Input: dimensioned drawing with shaded views. Units: mm. Origin: part minimum x, y, z. Round coordinates to 2 decimals unless told otherwise and drop trailing zeros. Loops run counter-clockwise (first coordinate to the right, second up) from the corner with the lowest first, then second, coordinate; pieces in that order, holes last. Notation, with made-up numbers: M 29,44 L 60,44 A20 cw 60,67 Z; hole C 56.5,62.5 d5. An arc over 180 degrees is marked long. Return JSON: item names as keys, results as strings.
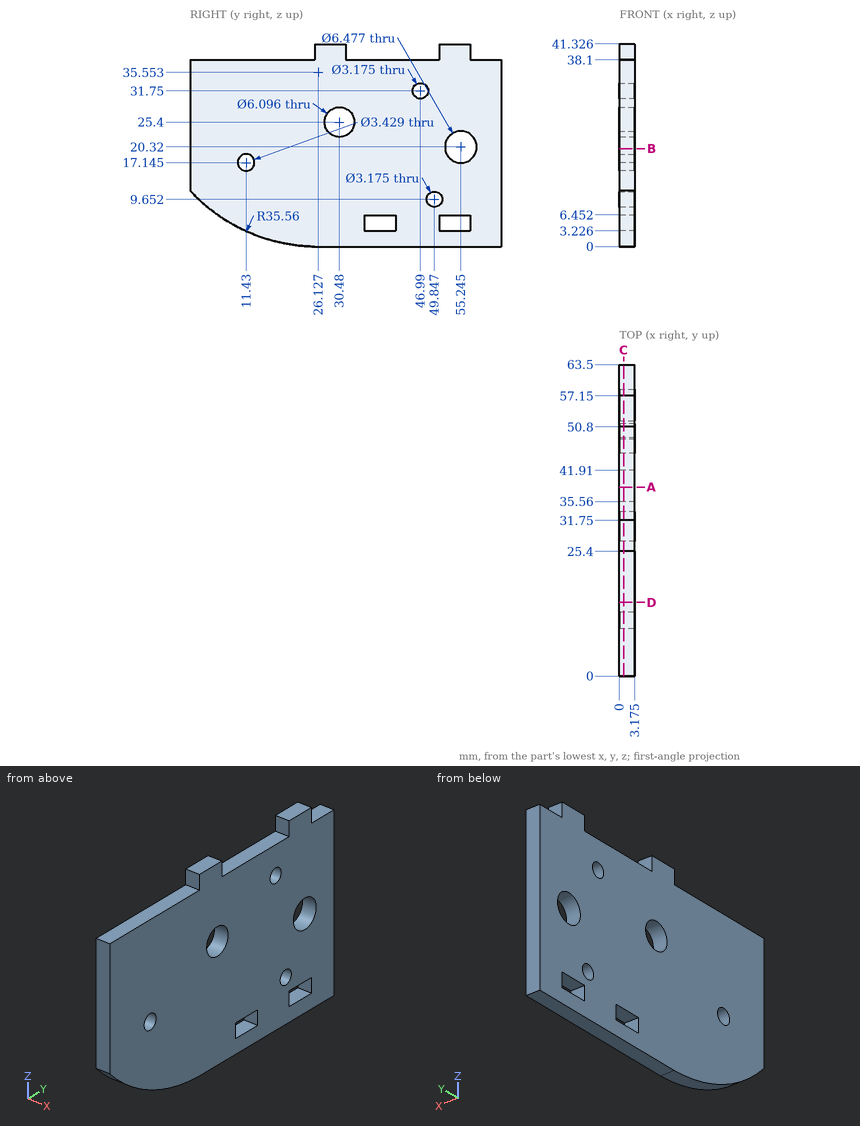
Q1. Section query C-C (x = 0.85). State how many separate pieces and enclosed holes the cut face has, plus the area to 3 significant figures.
Determined:
{"separate pieces": "1", "enclosed holes": "7", "area": "2,240 mm^2"}
Q2. Material intervals for L1, parallel to Y at x = 0.75, z = 31.75; L2, parallel to Y at x = 1.5, z = 17; L3, parallel to Z at x = 1.9, y = 31 (1 decimal), sorted ascending.
Determined:
{"L1": "y = 0 to 45.4, 48.58 to 63.5", "L2": "y = 0 to 9.72, 13.14 to 63.5", "L3": "z = 0 to 22.4, 28.4 to 41.3"}
Q3. Section query D-D (y = 15). Output: boundary loops of the cut face in (x, z) (1 decimal).
Determined:
{"outline": "M 0,1.8 L 3.2,1.8 L 3.2,38.1 L 0,38.1 Z"}
Q4. Section query B-B (z = 20). Output: boundary loops of the cut face in (x, y) (1 decimal).
Determined:
{"outline": "M 0,0 L 3.2,0 L 3.2,52 L 0,52 Z; M 0,58.5 L 3.2,58.5 L 3.2,63.5 L 0,63.5 Z"}
Q5. Pin query (flat end, axial travel): pin 1 (1.6 mm diameter, centred on x = 2, z = 40, fed in from -Y); pin 2 (1.6 mm diameter, centred on x = 1.5, y = 60.5, fed in from +Z). Return the tip coordinate at first contact, or that it passes through.
Determined:
{"pin 1": "stops at y = 25.4", "pin 2": "stops at z = 38.1"}
Q6. Section query A-A (y = 38.5). Output: boundary loops of the cut face in (x, z) (1 decimal).
Determined:
{"outline": "M 0,0 L 3.2,0 L 3.2,3.2 L 0,3.2 Z; M 0,6.5 L 3.2,6.5 L 3.2,38.1 L 0,38.1 Z"}
